Input: part model. Units: mm. Frame: model coordinates. A direction names the side the tool comes from. Coordinates: 2 decimals unless noted, no trailing zeros. Order: outer loops, then holes, each group sorted by start corner. A loop starts at its lowest first (then second) coordinate and runs counter-clockwise, first axis right, second up. Notation, with made-up numbers: (40, -24) - (48, -24) arc R33 cw to (48, 13) - close; hole circle Ø4 at (-2.5, -37). An arc over 180 degrees is marked (long way). One line per question, with ' | ' between items.
from build123d import *

# Parameters (mm, degrees)
BOSS_EXTRUDE1_DEPTH = 28
SKETCH3_W           = 16
SKETCH3_H           = 8
CUT_EXTRUDE1_DEPTH  = 12
SKETCH4_W           = 8
SKETCH4_H           = 16
CUT_EXTRUDE2_DEPTH  = 12
SKETCH5_W           = 16
SKETCH5_H           = 8
CUT_EXTRUDE3_DEPTH  = 12
SKETCH6_R           = 1.5
CUT_EXTRUDE4_DEPTH  = 21
CUT_EXTRUDE5_DEPTH  = 17
CUT_EXTRUDE6_DEPTH  = 6
CUT_EXTRUDE7_DEPTH  = 6
CIRPATTERN1_COUNT   = 3
SKETCH11_R          = 1
CUT_EXTRUDE8_DEPTH  = 10
CIRPATTERN2_COUNT   = 3
FILLET1_R           = 3.5


with BuildPart() as part:
    # Sketch1 → Boss-Extrude1 (new body)
    with BuildSketch(Plane.XY):
        Polygon((-45.033320997, -8), (-45.033320997, 8), (15.588457268, 43), (29.444863729, 35), (29.444863729, -35), (15.588457268, -43), align=None)
    extrude(amount=BOSS_EXTRUDE1_DEPTH)

    # Sketch3 → Cut-Extrude1 (cut)
    with BuildSketch(Plane(origin=(22.516660498, 39, 0), x_dir=(0.866025404, -0.5, 0), z_dir=(0.5, 0.866025404, 0))):
        with Locations((0, -4)):
            Rectangle(SKETCH3_W, SKETCH3_H)
    extrude(amount=-CUT_EXTRUDE1_DEPTH, mode=Mode.SUBTRACT)

    # Sketch4 → Cut-Extrude2 (cut)
    with BuildSketch(Plane.ZY.offset(45.033320997)):
        with Locations((4, 0)):
            Rectangle(SKETCH4_W, SKETCH4_H)
    extrude(amount=-CUT_EXTRUDE2_DEPTH, mode=Mode.SUBTRACT)

    # Sketch5 → Cut-Extrude3 (cut)
    with BuildSketch(Plane(origin=(22.516660498, -39, 0), x_dir=(0.866025404, 0.5, 0), z_dir=(0.5, -0.866025404, 0))):
        with Locations((0, 4)):
            Rectangle(SKETCH5_W, SKETCH5_H)
    extrude(amount=-CUT_EXTRUDE3_DEPTH, mode=Mode.SUBTRACT)

    # Sketch6 → Cut-Extrude4 (cut, through all)
    with BuildSketch(Plane(origin=(0, 0, 8), x_dir=(-1, 0, 0), z_dir=(0, 0, -1))):
        with Locations((-18.266660498, -31.638784068)):
            Circle(SKETCH6_R)
        with Locations((-18.266660498, 31.638784068)):
            Circle(SKETCH6_R)
        with Locations((36.533320997, 0)):
            Circle(SKETCH6_R)
    extrude(amount=-CUT_EXTRUDE4_DEPTH, mode=Mode.SUBTRACT)

    # Sketch7 → Cut-Extrude5 (cut)
    with BuildSketch(Plane.XY.offset(28)):
        Polygon((-42.033320997, -6.267949192), (-42.033320997, 6.267949192), (15.588457268, 39.535898385), (26.444863729, 33.267949192), (26.444863729, -33.267949192), (15.588457268, -39.535898385), align=None)
    extrude(amount=-CUT_EXTRUDE5_DEPTH, mode=Mode.SUBTRACT)

    # Sketch8 → Cut-Extrude6 (cut)
    with BuildSketch(Plane.XY.offset(11)):
        Polygon((-11.21880666, -23.805784253), (-21.750841765, -2.24015798), (-10.069460868, 3.464694369), (0.462574238, -18.100931904), align=None)
    cut_extrude6 = extrude(amount=-CUT_EXTRUDE6_DEPTH, mode=Mode.SUBTRACT)

    # Sketch9 → Cut-Extrude7 (cut, through all)
    with BuildSketch(Plane.XY.offset(5)):
        Polygon((-19.556667785, -6.732996787), (-7.875286887, -1.028144438), (-6.119947703, -4.622415484), (-17.801328601, -10.327267832), align=None)
    cut_extrude7 = extrude(amount=-CUT_EXTRUDE7_DEPTH, mode=Mode.SUBTRACT)

    # CirPattern1: Cut-Extrude6, Cut-Extrude7 ×3 about axis
    cirpattern1_axis = Axis((0, 0, 0), (0, 0, 1))
    for i in range(1, CIRPATTERN1_COUNT):
        add(cut_extrude6.rotate(cirpattern1_axis, i * 360 / CIRPATTERN1_COUNT), mode=Mode.SUBTRACT)
        add(cut_extrude7.rotate(cirpattern1_axis, i * 360 / CIRPATTERN1_COUNT), mode=Mode.SUBTRACT)

    # Sketch11 → Cut-Extrude8 (cut)
    with BuildSketch(Plane.ZY.offset(33.033320997)):
        with Locations((4.5, 4.25)):
            Circle(SKETCH11_R)
        with Locations((4.5, -4.25)):
            Circle(SKETCH11_R)
    cut_extrude8 = extrude(amount=-CUT_EXTRUDE8_DEPTH, mode=Mode.SUBTRACT)

    # CirPattern2: Cut-Extrude8 ×3 about axis
    cirpattern2_axis = Axis((0, 0, 0), (0, 0, 1))
    for i in range(1, CIRPATTERN2_COUNT):
        add(cut_extrude8.rotate(cirpattern2_axis, i * 360 / CIRPATTERN2_COUNT), mode=Mode.SUBTRACT)

    # Fillet1
    fillet1_edges = [part.edges().sort_by_distance(p)[0] for p in [
        (-14.722431864, 25.5, 0),
        (29.444863729, 0, 0),
        (-14.722431864, -25.5, 0),
    ]]
    fillet(fillet1_edges, radius=FILLET1_R)


solid = part.part
Item 1: Access query for faces 4 (the face through (-14.298, -25.745, 15.578)), 5 (the face through (-33.033, 0, 4)), 6 (the face through (0, -8, 11)), 7 (the face through (9.84, 26.77, 3.71)), 8 (the face through (26.5, 29.9, 4.1)). Directions: +Z, -Z, +X, -X, +Y, -Y. A direction counts if a zero-diameter tool reaches every point of the face in a straight line with its end or side. Return the directions, or none.
Data:
face 4: +Z, -Z, -X, -Y | face 5: -Z, -X | face 6: +Z | face 7: none | face 8: -Z, +Y
Item 2: Section C-C on x = -31.5. Count the separate pieces of the cut face and the enclosed holes in it, and give its area (3 significant figures).
Data:
separate pieces: 1 | enclosed holes: 2 | area: 453 mm^2
Item 3: Contact query for flat-ended pins moving along their axis: P1, Ø1.5, axis at x = -25.5, z = 3, coming from the +Y side; P2, Ø3, axis at x = -19.5, y = -4.5, coming from the +Z side; P3, Ø3.5, axis at x = 10.5, y = -12.5, coming from the +Z side; P4, Ø2.5, axis at x = 18.27, y = 31.64, coming from the +Z side. Output: stop coordinate, or through.
Data:
P1: y = 19.68 | P2: z = 11 | P3: z = 5 | P4: through
Item 4: Ray query, line 1 (X direction, y = -1.5, z = 24); line 2 (X direction, y = -10, z = 5.5); line 3 (Y direction, x = -26.25, z = 4.5). Return the intervals inside material, ascending.
Data:
line 1: -45.03 to -42.03, 26.44 to 29.44 | line 2: -41.57 to -17.96, -3.49 to 2.34, 18.01 to 29.44 | line 3: -18.84 to -5.25, -3.25 to 3.25, 5.25 to 18.84
Item 5: Draft query along Z for faces 1 (the face through (-39, 8, 4)), 2 (the face through (-8, 14, 5)), 3 (the face through (16.887, 22.701, 4.283)). Return one class per face: released by +Z, released by -Z, zero draft, split by the parting line, or undercut.
Data:
face 1: zero draft | face 2: released by +Z | face 3: undercut
Item 6: Section A-A on z = 21. Return the cut outline in (x, y).
Data:
outline: (-45.03, -8) - (15.59, -43) - (29.44, -35) - (29.44, 35) - (15.59, 43) - (-45.03, 8) - close; hole (-42.03, -6.27) - (15.59, -39.54) - (26.44, -33.27) - (26.44, 33.27) - (15.59, 39.54) - (-42.03, 6.27) - close
Item 7: Section B-B on y = 0. Return the cut outline in (x, z), and give its area (3 significant figures).
Data:
outline: (-45.03, 8) - (-38.03, 8) - (-38.03, 11) - (-42.03, 11) - (-42.03, 28) - (-45.03, 28) - close; (-35.03, 8) - (-33.03, 8) - (-33.03, 0) - (25.94, 0) arc R3.5 ccw to (29.44, 3.5) - (29.44, 28) - (26.44, 28) - (26.44, 11) - (24.75, 11) - (24.75, 5) - (9.08, 5) - (9.08, 11) - (-8.38, 11) - (-8.38, 5) - (-17.16, 5) - (-17.16, 11) - (-35.03, 11) - close | area: 667 mm^2
